```python
from build123d import *

# Parameters (mm, degrees)
BOSS_EXTRUDE1_DEPTH = 40
SKETCH8_W           = 40
SKETCH8_H           = 35
BOSS_EXTRUDE2_DEPTH = 1.5
SKETCH9_W           = 40
SKETCH9_H           = 35
BOSS_EXTRUDE3_DEPTH = 1.5
SKETCH11_R          = 1.5
CUT_EXTRUDE1_DEPTH  = 3.75
SKETCH12_R          = 1.5
CUT_EXTRUDE2_DEPTH  = 3.75
SKETCH4_W           = 20
SKETCH4_H           = 20
CUT_EXTRUDE3_DEPTH  = 4.5
CUT_EXTRUDE4_DEPTH  = 4.5
BOSS_EXTRUDE5_DEPTH = 40
SKETCH15_W          = 40
SKETCH15_H          = 10.404209308
SKETCH15_R          = 1.5
SKETCH15_W_2        = 30
SKETCH15_H_2        = 2.5
BOSS_EXTRUDE6_DEPTH = 2
SKETCH15_2_W        = 30
SKETCH15_2_H        = 2.5
CUT_EXTRUDE5_DEPTH  = 2.906774
SKETCH15_3_R        = 1.5
CUT_EXTRUDE6_DEPTH  = 2.156774
SKETCH17_W          = 40
SKETCH17_H          = 10.404209308
SKETCH17_R          = 1.5
SKETCH17_W_2        = 30
SKETCH17_H_2        = 2.5
BOSS_EXTRUDE7_DEPTH = 2
SKETCH17_2_R        = 1.5
CUT_EXTRUDE7_DEPTH  = 2.156774
SKETCH17_4_W        = 30
SKETCH17_4_H        = 2.5
CUT_EXTRUDE9_DEPTH  = 2.906774
FILLET1_R           = 1.5


with BuildPart() as part:
    # Sketch2 → Boss-Extrude1 (new body)
    with BuildSketch(Plane.XY):
        with BuildLine():
            Line((-67.116221114, 33.472568819), (-44.618654775, 60.284124329))
            ThreePointArc((-44.618654775, 60.284124329), (0, 75), (44.618654775, 60.284124329))
            Line((44.618654775, 60.284124329), (67.116221114, 33.472568819))
            ThreePointArc((67.116221114, 33.472568819), (67.449471383, 32.795865748), (67.77589897, 32.115845292))
            Line((67.77589897, 32.115845292), (65.142767665, 30.868126871))
            ThreePointArc((65.142767665, 30.868126871), (64.981306989, 31.206588688), (64.818087785, 31.54420599))
            Line((64.818087785, 31.54420599), (42.320521446, 58.3557615))
            ThreePointArc((42.320521446, 58.3557615), (0, 72.086208359), (-42.320521446, 58.3557615))
            Line((-42.320521446, 58.3557615), (-64.818087785, 31.54420599))
            ThreePointArc((-64.818087785, 31.54420599), (-64.981306989, 31.206588688), (-65.142767665, 30.868126871))
            Line((-65.142767665, 30.868126871), (-67.77589897, 32.115845292))
            ThreePointArc((-67.77589897, 32.115845292), (-67.449471383, 32.795865748), (-67.116221114, 33.472568819))
        make_face()
    extrude(amount=BOSS_EXTRUDE1_DEPTH)

    # Sketch8 → Boss-Extrude2 (add)
    with BuildSketch(Plane(origin=(-55.867437945, 46.878346574, 0), x_dir=(0, 0, 1), z_dir=(-0.766044443, 0.64278761, 0))):
        with Locations((20, 0)):
            Rectangle(SKETCH8_W, SKETCH8_H)
    extrude(amount=BOSS_EXTRUDE2_DEPTH)

    # Sketch9 → Boss-Extrude3 (add)
    with BuildSketch(Plane(origin=(55.867437945, 46.878346574, 0), x_dir=(0, 0, -1), z_dir=(0.766044443, 0.64278761, 0))):
        with Locations((-20, 0)):
            Rectangle(SKETCH9_W, SKETCH9_H)
    extrude(amount=BOSS_EXTRUDE3_DEPTH)

    # Sketch11 → Cut-Extrude1 (cut)
    with BuildSketch(Plane(origin=(-57.016504609, 47.842527989, 0), x_dir=(0, 0, 1), z_dir=(-0.766044443, 0.64278761, 0))):
        with Locations((37.39, 14.405)):
            Circle(SKETCH11_R)
        with Locations((2.61, 14.405)):
            Circle(SKETCH11_R)
        with Locations((2.61, -14.405)):
            Circle(SKETCH11_R)
        with Locations((37.39, -14.405)):
            Circle(SKETCH11_R)
    extrude(amount=-CUT_EXTRUDE1_DEPTH, mode=Mode.SUBTRACT)

    # Sketch12 → Cut-Extrude2 (cut)
    with BuildSketch(Plane(origin=(57.016504609, 47.842527989, 58.957611892), x_dir=(0.413175911, -0.492403877, -0.766044443), z_dir=(0.766044443, 0.64278761, 0))):
        with Locations((25.781104759, 2.828523492)):
            Circle(SKETCH12_R)
        with Locations((52.42413049, 25.184676556)):
            Circle(SKETCH12_R)
        with Locations((33.905419455, 47.254416963)):
            Circle(SKETCH12_R)
        with Locations((7.262393724, 24.898263898)):
            Circle(SKETCH12_R)
    extrude(amount=-CUT_EXTRUDE2_DEPTH, mode=Mode.SUBTRACT)

    # Sketch4 → Cut-Extrude3 (cut)
    with BuildSketch(Plane(origin=(-53.569304615, 44.949983745, 0), x_dir=(0, 0, -1), z_dir=(0.766044443, -0.64278761, 0))):
        with Locations((-20, 0)):
            Rectangle(SKETCH4_W, SKETCH4_H)
    extrude(amount=-CUT_EXTRUDE3_DEPTH, mode=Mode.SUBTRACT)

    # Sketch7 → Cut-Extrude4 (cut)
    with BuildSketch(Plane(origin=(53.569304615, 44.949983745, -58.957611892), x_dir=(0.413175911, -0.492403877, 0.766044443), z_dir=(-0.766044443, -0.64278761, 0))):
        Polygon((59.252471497, 36.664654087), (74.57336036, 49.52040628), (61.717608166, 64.841295143), (46.396719304, 51.985542949), align=None)
    extrude(amount=-CUT_EXTRUDE4_DEPTH, mode=Mode.SUBTRACT)

    # Sketch14 → Boss-Extrude5 (add)
    with BuildSketch(Plane.XY):
        Polygon((-68.787763199, 21.556091242), (-71.568228616, 22.427408515), (-67.77589897, 32.115845292), (-65.142767665, 30.868126871), align=None)
        Polygon((68.787763199, 21.556091242), (65.142767665, 30.868126871), (67.77589897, 32.115845292), (71.568228616, 22.427408515), align=None)
    extrude(amount=BOSS_EXTRUDE5_DEPTH)

    # Sketch15 → Boss-Extrude6 (add)
    with BuildSketch(Plane(origin=(-69.672063793, 27.271626904, 0), x_dir=(0, 0, -1), z_dir=(0.931203563, -0.364499553, 0))):
        with Locations((-20, 0)):
            Rectangle(SKETCH15_W, SKETCH15_H)
        with Locations((-37.5, 0)):
            Circle(SKETCH15_R, mode=Mode.SUBTRACT)
        with Locations((-2.5, 0)):
            Circle(SKETCH15_R, mode=Mode.SUBTRACT)
        with Locations((-20, 0)):
            Rectangle(SKETCH15_W_2, SKETCH15_H_2, mode=Mode.SUBTRACT)
    extrude(amount=-BOSS_EXTRUDE6_DEPTH)

    # Sketch15<2> → Cut-Extrude5 (cut)
    with BuildSketch(Plane(origin=(-69.672063793, 27.271626904, 0), x_dir=(0, 0, -1), z_dir=(0.931203563, -0.364499553, 0))):
        with Locations((-20, 0)):
            Rectangle(SKETCH15_2_W, SKETCH15_2_H)
    extrude(amount=CUT_EXTRUDE5_DEPTH, mode=Mode.SUBTRACT)

    # Sketch15<3> → Cut-Extrude6 (cut)
    with BuildSketch(Plane(origin=(-69.672063793, 27.271626904, 0), x_dir=(0, 0, -1), z_dir=(0.931203563, -0.364499553, 0))):
        with Locations((-37.5, 0)):
            Circle(SKETCH15_3_R)
        with Locations((-2.5, 0)):
            Circle(SKETCH15_3_R)
    extrude(amount=CUT_EXTRUDE6_DEPTH, mode=Mode.SUBTRACT)

    # Sketch17 → Boss-Extrude7 (add)
    with BuildSketch(Plane(origin=(69.672063793, 27.271626904, 0), x_dir=(0, 0, 1), z_dir=(-0.931203563, -0.364499553, 0))):
        with Locations((20, 0)):
            Rectangle(SKETCH17_W, SKETCH17_H)
        with Locations((2.5, 0)):
            Circle(SKETCH17_R, mode=Mode.SUBTRACT)
        with Locations((37.5, 0)):
            Circle(SKETCH17_R, mode=Mode.SUBTRACT)
        with Locations((20, 0)):
            Rectangle(SKETCH17_W_2, SKETCH17_H_2, mode=Mode.SUBTRACT)
    extrude(amount=-BOSS_EXTRUDE7_DEPTH)

    # Sketch17<2> → Cut-Extrude7 (cut)
    with BuildSketch(Plane(origin=(69.672063793, 27.271626904, 0), x_dir=(0, 0, 1), z_dir=(-0.931203563, -0.364499553, 0))):
        with Locations((37.5, 0)):
            Circle(SKETCH17_2_R)
        with Locations((2.5, 0)):
            Circle(SKETCH17_2_R)
    extrude(amount=CUT_EXTRUDE7_DEPTH, mode=Mode.SUBTRACT)

    # Sketch17<4> → Cut-Extrude9 (cut)
    with BuildSketch(Plane(origin=(69.672063793, 27.271626904, 0), x_dir=(0, 0, 1), z_dir=(-0.931203563, -0.364499553, 0))):
        with Locations((20, 0)):
            Rectangle(SKETCH17_4_W, SKETCH17_4_H)
    extrude(amount=CUT_EXTRUDE9_DEPTH, mode=Mode.SUBTRACT)

    # Fillet1
    fillet1_edges = [part.edges().sort_by_distance(p)[0] for p in [
        (-68.787763199, 21.556091242, 20),
        (68.787763199, 21.556091242, 20),
        (-71.990095361, 26.836621557, 20),
        (-71.078846477, 29.164630464, 20),
        (-67.42088993, 25.048104625, 20),
        (-66.509641046, 27.376113532, 20),
        (71.078846477, 29.164630464, 20),
        (71.990095361, 26.836621557, 20),
        (66.509641046, 27.376113532, 20),
        (67.42088993, 25.048104625, 20),
    ]]
    fillet(fillet1_edges, radius=FILLET1_R)


solid = part.part
```
Source: CAD feature listing. Evaluate the final solid. Frame: model axes, mm. A direction names the side the tool comes from. Coordinates: 2 decimals unless noted, no trailing zeros. Write each loop counter-clockwise with the first axis right and the second up, starting at its lowest first coordinate (ties: lowest second). Pieces come first, ordered by that corner, then holes. Notation, with made-up numbers: M 14,-9 L 23,-9 A27 cw 23,10 Z; hole C -4.75,30.25 d9. An arc over 180 degrees is marked long. Answer as a JSON object with one key per item and string values.
1. Ray query, L1, parallel to X at y = 38.5, z = 19.5; L2, parallel to X at y = 40, z = 8; L3, parallel to Y at x = 2.5, z = 34. Return the intervals inside material, ascending.
Evaluation:
{"L1": "-64.86 to -61.44, 61.44 to 64.86", "L2": "-63.6 to -57.72, 57.72 to 63.6", "L3": "72.04 to 74.96"}
2. Access query for faces 4 (the flat face through (-70.244, 31.298, 20.28)), 5 (the flat face through (48.8, 54, 20.1)), 6 (the flat face through (-69, 27, 5)), 7 (the flat face through (-60.91, 36.2, 19.72)). Directions: +Z, -Z, +X, -X, +Y, -Y. A direction counts if a zero-diameter tool reaches every point of the face in a straight line with its end or side. Return the directions, or none.
Evaluation:
{"face 4": "+Z, -Z, -X, +Y", "face 5": "+X, -Y", "face 6": "none", "face 7": "+Z, -Z, -Y"}
3. Cut plane C-C on x = -23. Output: boundary loops of the cut face in (y, z), plus the area to 3 significant figures.
Evaluation:
{"outline": "M 68.32,0 L 71.39,0 L 71.39,40 L 68.32,40 Z", "area": "123 mm^2"}
4. Contact query for flat-ended pins moving along their axis: P1, Ø5, axis at y = 50.5, z = 26.5, coming from the -X side; P2, Ø18, axis at x = -55.5, y = 49.5, coming from the -Z side; P3, Ø2, axis at x = 1.5, z = 22, coming from the +Y side; P4, Ø10, axis at x = 39, z = 9, coming from the +Y side. Output: stop coordinate, or through.
Evaluation:
{"P1": "x = -47.61", "P2": "z = 0", "P3": "y = 75", "P4": "y = 66.85"}
5. Draft query along Y for faces 1 (the flat face through (61.7, 38.72, 19.86)), 2 (the flat face through (46.228, 53.699, 19.72)), 3 (the cylindrical face through (-47.282, 56.567, 2.285)). Return one class per face: released by +Y, released by -Y, zero draft, split by the parting line, or undercut.
Evaluation:
{"face 1": "released by +Y", "face 2": "released by -Y", "face 3": "undercut"}
6. Cut plane B-B on y = 44. Output: boundary loops of the cut face in (x, z).
Evaluation:
{"outline": "M -60.24,0 L -54.37,0 L -54.37,10 L -60.24,10 Z; M -60.24,30 L -54.37,30 L -54.37,40 L -60.24,40 Z; M 54.37,0 L 60.24,0 L 60.24,10 L 54.37,10 Z; M 54.37,30 L 60.24,30 L 60.24,40 L 54.37,40 Z"}
7. Cut plane A-A on y = 68. Output: boundary loops of the cut face in (x, z), plus the area to 3 significant figures.
Evaluation:
{"outline": "M -31.64,0 L -23.93,0 L -23.93,40 L -31.64,40 Z; M 23.93,0 L 31.64,0 L 31.64,40 L 23.93,40 Z", "area": "617 mm^2"}
8. Cut plane D-D on z = 24. State how many separate pieces and enclosed holes the cut face has, plus the area to 3 significant figures.
Evaluation:
{"separate pieces": "5", "enclosed holes": "0", "area": "484 mm^2"}
